from build123d import *

# Parameters (mm, degrees)
SKIZZE1_W                             = 49
SKIZZE1_H                             = 49
AUFSATZ_LINEAR_AUSTRAGEN1_DEPTH       = 11.5
SKIZZE2_W                             = 42.3
SKIZZE2_H                             = 42.3
SCHNITT_LINEAR_AUSTRAGEN1_DEPTH       = 5
SKIZZE3_R                             = 2.85
SCHNITT_LINEAR_AUSTRAGEN2_DEPTH       = 7
AUFSATZ_LINEAR_AUSTRAGEN2_DEPTH       = 2
AUFSATZ_LINEAR_AUSTRAGEN2_DEPTH_BACK  = 5
SKIZZE6_W                             = 42.3
SKIZZE6_H                             = 42.3
SCHNITT_LINEAR_AUSTRAGEN3_DEPTH       = 7
AUFSATZ_LINEAR_START                  = 18
SKIZZE8_R                             = 7.5
AUFSATZ_LINEAR_AUSTRAGEN3_DEPTH       = 18
FASE2_SIZE                            = 10
FASE4_SIZE                            = 1
FASE4_SIZE2                           = 0.577350269
SKIZZE17_R                            = 3
SCHNITT_LINEAR_AUSTRAGEN8_DEPTH       = 23
SKIZZE18_R                            = 11.25
SCHNITT_LINEAR_AUSTRAGEN9_DEPTH       = 2.2
SCHNITT_LINEAR_AUSTRAGEN10_DEPTH      = 64.402786508
SCHNITT_LINEAR_AUSTRAGEN10_DEPTH_BACK = 64.402786508
SKIZZE10_R                            = 2.5
SKIZZE19_R                            = 4.4
SCHNITT_LINEAR_AUSTRAGEN11_DEPTH      = 12
KREISMUSTER1_COUNT                    = 3
SKIZZE21_R                            = 1.5
SCHNITT_LINEAR_AUSTRAGEN12_DEPTH      = 10
SKIZZE22_R                            = 3
SCHNITT_LINEAR_AUSTRAGEN13_DEPTH      = 2


with BuildPart() as part:
    # Skizze1 → Aufsatz-Linear austragen1 (new body)
    with BuildSketch(Plane.XY):
        Rectangle(SKIZZE1_W, SKIZZE1_H)
    extrude(amount=AUFSATZ_LINEAR_AUSTRAGEN1_DEPTH)

    # Skizze2 → Schnitt-Linear austragen1 (cut)
    with BuildSketch(Plane.XY.offset(11.5)):
        Rectangle(SKIZZE2_W, SKIZZE2_H)
    extrude(amount=-SCHNITT_LINEAR_AUSTRAGEN1_DEPTH, mode=Mode.SUBTRACT)

    # Skizze3 → Schnitt-Linear austragen2 (cut)
    with BuildSketch(Plane.XY.offset(6.5)):
        Circle(SKIZZE3_R)
    extrude(amount=-SCHNITT_LINEAR_AUSTRAGEN2_DEPTH, mode=Mode.SUBTRACT)

    # Skizze5 → Aufsatz-Linear austragen2 (add, two sides: drawn at the far end of the back side and taken through both)
    with BuildSketch(Plane.XY.offset(6.5).offset(-AUFSATZ_LINEAR_AUSTRAGEN2_DEPTH_BACK)):
        with BuildLine():
            Line((26.560889132, 23.995190528), (0, 8.660254038))
            Line((0, 8.660254038), (-26.560889132, 23.995190528))
            ThreePointArc((-26.560889132, 23.995190528), (-36.806079661, 21.25), (-34.060889132, 11.004809472))
            Line((-34.060889132, 11.004809472), (-7.5, -4.330127019))
            Line((-7.5, -4.330127019), (-7.5, -35))
            ThreePointArc((-7.5, -35), (0, -42.5), (7.5, -35))
            Line((7.5, -35), (7.5, -4.330127019))
            Line((7.5, -4.330127019), (34.060889132, 11.004809472))
            ThreePointArc((34.060889132, 11.004809472), (36.806079661, 21.25), (26.560889132, 23.995190528))
        make_face()
    extrude(amount=AUFSATZ_LINEAR_AUSTRAGEN2_DEPTH + AUFSATZ_LINEAR_AUSTRAGEN2_DEPTH_BACK)

    # Skizze6 → Schnitt-Linear austragen3 (cut)
    with BuildSketch(Plane.XY.offset(11.5)):
        Rectangle(SKIZZE6_W, SKIZZE6_H)
    extrude(amount=-SCHNITT_LINEAR_AUSTRAGEN3_DEPTH, mode=Mode.SUBTRACT)

    # Skizze8 → Aufsatz-Linear austragen3 (add)
    with BuildSketch(Plane(origin=(0, 0, 1.5), x_dir=(-1, 0, 0), z_dir=(0, 0, -1)).offset(AUFSATZ_LINEAR_START)):
        with Locations(Location((-30.310889132, 17.5, 0), (0, 0, 240))):
            Circle(SKIZZE8_R)
        with Locations((0, -35)):
            Circle(SKIZZE8_R)
        with Locations((30.310889132, 17.5)):
            Circle(SKIZZE8_R)
    extrude(amount=-AUFSATZ_LINEAR_AUSTRAGEN3_DEPTH)

    # Fase2
    fase2_edges = [part.edges().sort_by_distance(p)[0] for p in [
        (-24.5, 5.484827557, 5),
        (-7.5, -24.5, 5),
        (7.5, -24.5, 5),
        (24.5, 5.484827557, 5),
    ]]
    chamfer(fase2_edges, length=FASE2_SIZE)

    # Fase4
    fase4_edges = [part.edges().sort_by_distance(p)[0] for p in [
        (21.15, 0, 11.5),
        (0, 21.15, 11.5),
        (-21.15, 0, 11.5),
        (0, -21.15, 11.5),
    ]]
    fase4_side = [part.faces().sort_by_distance(p)[0] for p in [
        (0, 23.807035354, 11.5),
    ]]
    chamfer(fase4_edges, length=FASE4_SIZE, length2=FASE4_SIZE2, reference=fase4_side[0])

    # Skizze17 → Schnitt-Linear austragen8 (cut)
    with BuildSketch(Plane.XY.offset(4.5)):
        Circle(SKIZZE17_R)
    extrude(amount=-SCHNITT_LINEAR_AUSTRAGEN8_DEPTH, mode=Mode.SUBTRACT)

    # Skizze18 → Schnitt-Linear austragen9 (cut)
    with BuildSketch(Plane.XY.offset(4.5)):
        Circle(SKIZZE18_R)
    extrude(amount=-SCHNITT_LINEAR_AUSTRAGEN9_DEPTH, mode=Mode.SUBTRACT)

    # Skizze10 → Schnitt-Linear austragen10 (cut, two sides: drawn at the far end of the back side and taken through both)
    with BuildSketch(Plane(origin=(0, 0, -16.5), x_dir=(-1, 0, 0), z_dir=(0, 0, -1)).offset(-SCHNITT_LINEAR_AUSTRAGEN10_DEPTH_BACK)):
        with Locations((-30.310889132, 17.5)):
            Circle(SKIZZE10_R)
        with Locations((30.310889132, 17.5)):
            Circle(SKIZZE10_R)
        with Locations((0, -35)):
            Circle(SKIZZE10_R)
    extrude(amount=SCHNITT_LINEAR_AUSTRAGEN10_DEPTH + SCHNITT_LINEAR_AUSTRAGEN10_DEPTH_BACK, mode=Mode.SUBTRACT)

    # Skizze19 → Schnitt-Linear austragen11 (cut)
    with BuildSketch(Plane.XY.offset(8.5)):
        with Locations((30.310889132, 17.5)):
            Circle(SKIZZE19_R)
    schnitt_linear_austragen11 = extrude(amount=-SCHNITT_LINEAR_AUSTRAGEN11_DEPTH, mode=Mode.SUBTRACT)

    # Kreismuster1: Schnitt-Linear austragen11 ×3 about axis
    kreismuster1_axis = Axis((0, 0, 0), (0, 0, 1))
    for i in range(1, KREISMUSTER1_COUNT):
        add(schnitt_linear_austragen11.rotate(kreismuster1_axis, i * 360 / KREISMUSTER1_COUNT), mode=Mode.SUBTRACT)

    # Skizze21 → Schnitt-Linear austragen12 (cut)
    with BuildSketch(Plane.XY.offset(4.5)):
        with Locations((-15, 15.5)):
            Circle(SKIZZE21_R)
        with Locations((15, 15.5)):
            Circle(SKIZZE21_R)
        with Locations((15, -15.5)):
            Circle(SKIZZE21_R)
        with Locations((-15, -15.5)):
            Circle(SKIZZE21_R)
    extrude(amount=-SCHNITT_LINEAR_AUSTRAGEN12_DEPTH, mode=Mode.SUBTRACT)

    # Skizze22 → Schnitt-Linear austragen13 (cut)
    with BuildSketch(Plane(origin=(0, 0, 0), x_dir=(-1, 0, 0), z_dir=(0, 0, -1))):
        with Locations((-15, 15.5)):
            Circle(SKIZZE22_R)
        with Locations((15, 15.5)):
            Circle(SKIZZE22_R)
        with Locations((15, -15.5)):
            Circle(SKIZZE22_R)
        with Locations((-15, -15.5)):
            Circle(SKIZZE22_R)
    extrude(amount=-SCHNITT_LINEAR_AUSTRAGEN13_DEPTH, mode=Mode.SUBTRACT)


solid = part.part
Here's how the part is built. I have some questions about the finished solid (model axes, mm). A direction names the side the tool comes from. Coordinates: 2 decimals unless noted, no trailing zeros. Loops run counter-clockwise (first coordinate to the right, second up) from the corner with the lowest first, then second, coordinate; pieces in that order, holes last.
1. For P1, Ø4, axis at y = -3, z = 3, coming from the -X side; P2, Ø3.5, axis at y = -11.5, z = 6.5, coming from the -X side; P3, Ø3, axis at x = -9, y = 13.5, coming from the -Z side, each with a flat end and sliding along its axis, tell me the tip position at first contact or that it passes through.
2. Imagine slicing it at A-A, the plane x = 15. Count the separate pieces of the cut face and the enclosed holes in it, and give its area (3 significant figures).
3. Imagine slicing it at B-B, the plane x = 29. Please give me the cut outline in (y, z), and give its area (3 significant figures).
4. If we mould it in two halves opening along X, with no side actions, what happens to faces 1 (the cylindrical face through (13.5, 15.57, 3.27)), 2 (the flat face through (-30, 10, 8.5)), 3 (the flat face through (12, -30, 5))? For each: pulls with the +X half, pulls with the -X half, needs draft (parallel to the pull), parting line crosses it, or undercut.
5. For faces 4 (the flat face through (0, 24.5, 6)), 5 (the cylindrical face through (17.4, 13.7, 1)), 6 (the flat face through (-12, -30, 5)), 7 (the flat face through (0, -21.15, 8)), which set-ups out of +Z, -Z, +X, -X, +Y, -Y let a thin tool reach every point of the face, with its end or its side?
6. I need wall thicknesses on L1, parallel to Y at x = 15, z = 1.25; L2, parallel to X at y = -16.5, z = 0.5; L3, parallel to X at y = -30, z = 4.5. Which ranges of each line are inside material? Lowest first, please.
7. Imagine slicing it at C-C, the plane y = 0. Please give me the cut outline in (x, z), and give its area (3 significant figures).
Taken from the geometry:
1. P1: stops at x = -26.53
1. P2: stops at x = -24.5
1. P3: stops at z = 0
2. separate pieces: 3
2. enclosed holes: 0
2. area: 245 mm2
3. outline: (3.28, 1.5) - (10.12, 1.5) - (10.12, -16.5) - (15.37, -16.5) - (15.37, -3.5) - (13.3, -3.5) - (13.3, 8.5) - (3.28, 8.5) - close; (19.63, -16.5) - (24.88, -16.5) - (24.88, 8.5) - (21.7, 8.5) - (21.7, -3.5) - (19.63, -3.5) - close
3. area: 261 mm2
4. face 1: undercut
4. face 2: needs draft
4. face 3: pulls with the +X half
5. face 4: +Z, -Z, +Y
5. face 5: -Z
5. face 6: +Z, -Z, -X, -Y
5. face 7: +Z
6. L1: y = -24.5 to -18.5, -12.5 to 12.5, 18.5 to 24.5
6. L2: x = -24.5 to -17.83, -12.17 to 12.17, 17.83 to 24.5
6. L3: x = -12 to 12
7. outline: (-27.11, 1.5) - (-24.5, 1.5) - (-24.5, 0) - (-3, 0) - (-3, 2.3) - (-11.25, 2.3) - (-11.25, 4.5) - (-21.15, 4.5) - (-21.15, 10.92) - (-22.15, 11.5) - (-24.5, 11.5) - (-24.5, 8.5) - (-27.11, 8.5) - close; (3, 0) - (24.5, 0) - (24.5, 1.5) - (27.11, 1.5) - (27.11, 8.5) - (24.5, 8.5) - (24.5, 11.5) - (22.15, 11.5) - (21.15, 10.92) - (21.15, 4.5) - (11.25, 4.5) - (11.25, 2.3) - (3, 2.3) - close
7. area: 240 mm2
